from build123d import *
from build123d.topology import SkipClean

# Parameters (mm, degrees)
SKETCH2_R            = 6
BOSS_EXTRUDE1_DEPTH  = 14.5
CHAMFER1_SIZE        = 2
BOSS_EXTRUDE3_DEPTH  = 15.6
M4_CLEARANCE_HOLE1_D = 4.5
M4_CLEARANCE_HOLE2_D = 4.5


with BuildPart() as part:
    # Sketch2 → Boss-Extrude1 (new body)
    with BuildSketch(Plane(origin=(0, 0, 0), x_dir=(1, 0, 0), z_dir=(0, 1, 0))):
        with Locations(Location((0, 0, 0), (0, 0, 90))):
            Circle(SKETCH2_R)
    extrude(amount=BOSS_EXTRUDE1_DEPTH)

    # Chamfer1
    chamfer1_edges = [part.edges().sort_by_distance(p)[0] for p in [
        (0, 0, 6),
    ]]
    chamfer(chamfer1_edges, length=CHAMFER1_SIZE)

    # Sketch3 → Boss-Extrude3 (add)
    with SkipClean():  # the faces are left unmerged after this step: merging them gives an invalid solid
        with BuildSketch(Plane(origin=(0, 14.5, 0), x_dir=(1, 0, 0), z_dir=(0, 1, 0))):
            with BuildLine():
                Line((-2.85, 0), (-2.85, 5.279915))
                ThreePointArc((-2.85, 5.279915), (0, 6), (2.85, 5.279915))
                Line((2.85, 5.279915), (2.85, -5.279915))
                ThreePointArc((2.85, -5.279915), (0, -6), (-2.85, -5.279915))
                Line((-2.85, -5.279915), (-2.85, 0))
            make_face()
        extrude(amount=BOSS_EXTRUDE3_DEPTH)

    # M4 Clearance Hole1 (through all)
    with Locations(Plane.XY.offset(6)):
        with Locations((0, 6.2)):
            Hole(M4_CLEARANCE_HOLE1_D / 2)

    # M4 Clearance Hole2 (through all)
    with Locations(Plane(origin=(2.85, 0, 0), x_dir=(0, 0, -1), z_dir=(1, 0, 0))):
        with Locations((0, 21.1)):
            Hole(M4_CLEARANCE_HOLE2_D / 2)


solid = part.part
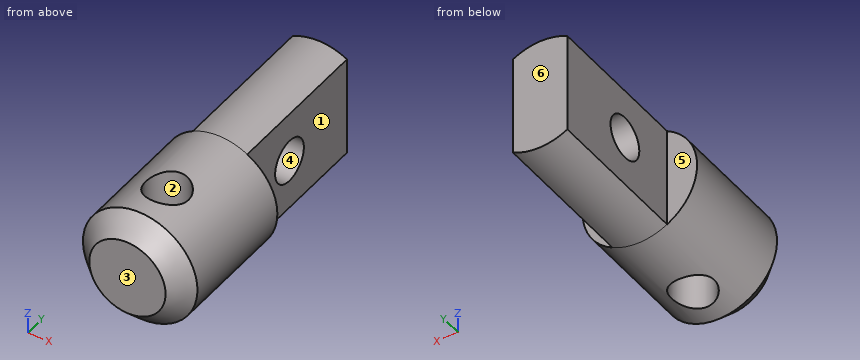
For this review, take the finished solid that the model builds, in its own axes (mm). Face numbers are marked on the shaded views. A direction names the side the tool comes from. Coordinates: 2 decimals unless noted, no trailing zeros. Loops run counter-clockwise (first coordinate to the right, second up) from the corner with the lowest first, then second, coordinate; pieces in that order, holes last. Notation, with made-up numbers: (74.25, -23) -> (79.25, -23) arc R35 ccw to (79.25, 15) -> close; hole circle Ø5 at (13.25, 42.25). An arc over 180 degrees is marked (long way). Write each question's results on one line, items separated by ' | '.
Q1. For pin 1 Ø1.5 at (y, z) = (7, -5) entering from +X; pin 2 Ø1 at (x, y) = (-4, 24.5) entering from +Z; pin 3 Ø2.5 at (x, z) = (-4.5, 1) entering from +Y; pin 4 Ø7 at (y, z) = (21.1, 0) entering from -X, all flat-tipped, find the tip position at first contact; note any pin that passes through.
Taken from the geometry:
pin 1: x = 4.24 | pin 2: through | pin 3: y = 14.5 | pin 4: x = -2.85
Q2. Mouldability with a two-part tool opening along Y and no side actions: class the marked faces 1, 2, 3 and 4 as +Y half, -Y half, draft (parallel to the pull), parting line (faces both ways), or undercut.
Taken from the geometry:
face 1: draft | face 2: undercut | face 3: -Y half | face 4: undercut
Q3. Machinability: for the marked faces 5 and 6, which of the approach directions +Z, -Z, +X, -X, +Y, -Y give a long, thin tool a straight path to every point of the face, cutting with its end or side? Answer none if there is none.
Taken from the geometry:
face 5: +Z, -Z, -X, +Y | face 6: +Z, -Z, +X, -X, +Y
Q4. Add section B-B, the plane z = 0. State the section outline as (x, y) points.
Taken from the geometry:
outline: (-6, 2) -> (-4, 0) -> (4, 0) -> (6, 2) -> (6, 14.5) -> (2.85, 14.5) -> (2.85, 18.85) -> (-2.85, 18.85) -> (-2.85, 14.5) -> (-6, 14.5) -> close; (-2.85, 23.35) -> (2.85, 23.35) -> (2.85, 30.1) -> (-2.85, 30.1) -> close; hole circle Ø4.5 at (0, 6.2)
Q5. Add section D-D, the plane y = 11.5. State the section outline as (x, z) points.
Taken from the geometry:
outline: circle Ø12 at (0, 0)
Q6. Add section A-A, the plane x = 0. State the section outline as (y, z) points.
Taken from the geometry:
outline: (0, -4) -> (2, -6) -> (3.95, -6) -> (3.95, 6) -> (2, 6) -> (0, 4) -> close; (8.45, -6) -> (30.1, -6) -> (30.1, 6) -> (8.45, 6) -> close; hole circle Ø4.5 at (21.1, 0)
Q7. Add section C-C, the plane y = 21.1. State the section outline as (x, z) points, then the cut area to 3 significant figures.
Taken from the geometry:
outline: (-2.85, -5.28) arc R6 ccw to (2.85, -5.28) -> (2.85, -2.25) -> (-2.85, -2.25) -> close; (-2.85, 2.25) -> (2.85, 2.25) -> (2.85, 5.28) arc R6 ccw to (-2.85, 5.28) -> close | area: 40.1 mm²
Q8. To check wall thickness, follow line 1 along Y through (x, z) = (0, 0.25); line 2 along Y through (x, z) = (0.8, 0); line 3 along Y through (x, z) = (0, -3.5). State the ranges of each line that lie inside material, in increasing order. Write a range as [from, to].
Taken from the geometry:
line 1: [0, 3.95], [8.45, 18.86], [23.34, 30.1] | line 2: [0, 4.1], [8.3, 18.85], [23.35, 30.1] | line 3: [0, 3.95], [8.45, 30.1]
